```python
from build123d import *

# Parameters (mm, degrees)
SKETCH1_R           = 1.5
BOSS_EXTRUDE1_DEPTH = 2


with BuildPart() as part:
    # Sketch1 → Boss-Extrude1 (new body)
    with BuildSketch(Plane.XY):
        with BuildLine():
            Line((-5.322767432, 19.832757644), (-4.500006862, -0.184957582))
            ThreePointArc((-4.500006862, -0.184957582), (-0.000167017, -4.503806283), (4.499993132, -0.185291335))
            Line((4.499993132, -0.185291335), (5.67721776, 19.814708665))
            ThreePointArc((5.67721776, 19.814708665), (8.148561948, 21.404983206), (10.180318916, 23.528301089))
            Line((10.180318916, 23.528301089), (12.180312779, 23.523346368))
            ThreePointArc((12.180312779, 23.523346368), (12.679597114, 23.812434692), (12.680312779, 24.389371772))
            Line((12.680312779, 24.389371772), (11.684612917, 26.123898158))
            ThreePointArc((11.684612917, 26.123898158), (11.934719035, 26.754030681), (12.150293859, 27.396796239))
            Line((12.150293859, 27.396796239), (14.031367948, 28.076178512))
            ThreePointArc((14.031367948, 28.076178512), (14.401667723, 28.518597977), (14.205016126, 29.060986265))
            Line((14.205016126, 29.060986265), (12.67612135, 30.350358501))
            ThreePointArc((12.67612135, 30.350358501), (12.695626208, 31.028030714), (12.678361511, 31.705763698))
            Line((12.678361511, 31.705763698), (14.213630529, 32.987539436))
            ThreePointArc((14.213630529, 32.987539436), (14.410282126, 33.529927724), (14.039982351, 33.972347189))
            Line((14.039982351, 33.972347189), (12.162299935, 34.661047954))
            ThreePointArc((12.162299935, 34.661047954), (11.948850959, 35.304522586), (11.700829119, 35.935478396))
            Line((11.700829119, 35.935478396), (12.705116964, 37.665046528))
            ThreePointArc((12.705116964, 37.665046528), (12.704401299, 38.241983607), (12.205116964, 38.531071932))
            Line((12.205116964, 38.531071932), (10.205123119, 38.536033749))
            ThreePointArc((10.205123119, 38.536033749), (9.784465406, 39.067698263), (9.335601516, 39.575774317))
            Line((9.335601516, 39.575774317), (9.687776253, 41.5445234))
            ThreePointArc((9.687776253, 41.5445234), (9.489779645, 42.086422145), (8.92173181, 42.18731101))
            Line((8.92173181, 42.18731101), (7.040655311, 41.507935412))
            ThreePointArc((7.040655311, 41.507935412), (6.463526388, 41.863663221), (5.867960059, 42.187578047))
            Line((5.867960059, 42.187578047), (5.525544216, 44.158047887))
            ThreePointArc((5.525544216, 44.158047887), (5.154147979, 44.59954731), (4.585851596, 44.500068031))
            Line((4.585851596, 44.500068031), (3.050578029, 43.21829774))
            ThreePointArc((3.050578029, 43.21829774), (2.386588163, 43.355182821), (1.716153483, 43.455867511))
            Line((1.716153483, 43.455867511), (0.720447466, 45.190390364))
            ThreePointArc((0.720447466, 45.190390364), (0.220447466, 45.47823912), (-0.279552534, 45.190390364))
            Line((-0.279552534, 45.190390364), (-1.283846517, 43.460825796))
            ThreePointArc((-1.283846517, 43.460825796), (-12.125641313, 33.154858755), (-5.322767432, 19.832757644))
        make_face()
        with Locations((0.19564328, 31.048690205)):
            Circle(SKETCH1_R, mode=Mode.SUBTRACT)
        with Locations((0, 38.546138017)):
            Circle(SKETCH1_R, mode=Mode.SUBTRACT)
        with Locations((0, 23.551242392)):
            Circle(SKETCH1_R, mode=Mode.SUBTRACT)
        Circle(SKETCH1_R, mode=Mode.SUBTRACT)
    extrude(amount=BOSS_EXTRUDE1_DEPTH)


solid = part.part
```
The model under review builds one solid part; all positions refer to its coordinate system, in mm. A direction names the side the tool comes from. Coordinates: 2 decimals unless noted, no trailing zeros. Write each loop counter-clockwise with the first axis right and the second up, starting at its lowest first coordinate (ties: lowest second). Pieces come first, ordered by that corner, then holes. Notation, with made-up numbers: (84.5, -16) - (96.5, -16) arc R13 cw to (96.5, -11) - close; hole circle Ø6 at (-19, 48.25). An arc over 180 degrees is marked (long way). Answer in a Markdown table with one row per item. Add a question column.
Q1. Consider section B-B on x = 7.5. Give the boundary of the cut face in (y, z).
Q2. Clearance check with flat-ended pins moving along their axes: pin 1 (5 mm diameter, centred on x = 0, y = 23.55, fed in from +Z); pin 2 (1 mm diameter, centred on y = 4, z = 0.5, fed in from +X); pin 3 (1 mm diameter, centred on y = 15.5, z = 1.5, fed in from +X). State where each tip first meets the part, or that it passes through.
Q3. For faces 1 (the face through (-0.097, -4.503, 0.986)), 2 (the face through (6.47, 41.86, 0.99)), 3 (the face through (13.078, 27.732, 0.986)), list the 3-axis set-ups (+Z, -Z, +X, -X, +Y, -Y) from which the entire face can be reached by the end or side of a thin tool; tool diameter is ignored.
Q4. Consider section A-A on z = 1.65. Give the number of separate pieces and of enclosed holes in the cut face, then the cut area to 3 significant figures.
Q5. To check wall thickness, follow line 1 along Y through (x, z) = (0, 0.55); line 2 along Y through (x, z) = (11.5, 1.4); line 3 along X through (y, z) = (-0.5, 0.55). State the ranges of each line that lie inside material, in increasing order. Write a range as from..to.
Q6. Consider section C-C on y = 15. Give the boundary of the cut face in (x, z).
Answers below:
| question | item | result |
|---|---|---|
| 1 | outline | (20.9, 0) - (41.67, 0) - (41.67, 2) - (20.9, 2) - close |
| 2 | pin 1 | z = 2 |
| 2 | pin 2 | x = 4.78 |
| 2 | pin 3 | x = 5.45 |
| 3 | face 1 | +Z, -Z, -Y |
| 3 | face 2 | +Z, -Z, +Y |
| 3 | face 3 | +Z, -Z, +X |
| 4 | separate pieces | 1 |
| 4 | enclosed holes | 4 |
| 4 | area | 708 mm² |
| 5 | line 1 | -4.5..-1.5, 1.5..22.05, 25.05..29.56, 32.54..37.05, 40.05..45.43 |
| 5 | line 2 | 23.53..38.53 |
| 5 | line 3 | -4.48..-1.41, 1.41..4.48 |
| 6 | outline | (-5.12, 0) - (5.39, 0) - (5.39, 2) - (-5.12, 2) - close |
